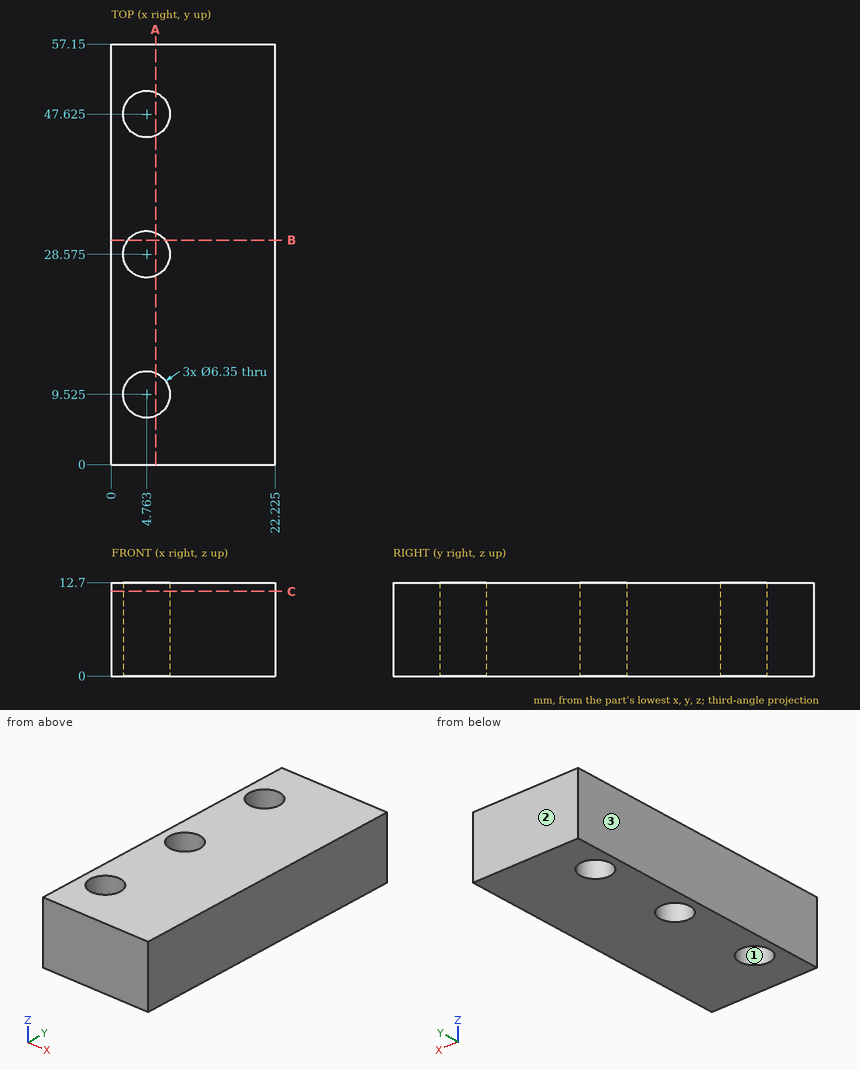
Design review of the part shown in the three views and the two pictorial views. Dimensions are in mm from the part's minimum x, y and z. Coordinates: 2 decimals unless noted, no trailing zeros. Order: outer loops, then holes, each group sorted by start corner. A loop starts at its lowest first (then second) coordinate and runs counter-clockwise, first axis right, second up.
Item 1: For line 1 (Y direction, x = 6.5, z = 4.75); line 2 (X direction, y = 27, z = 12) (1 decimal); line 3 (Y direction, x = 4, z = 7.75), list the stretches that pass through material, from the lowest coordinate up.
Item 2: Take a section at A-A, the plane x = 6. Write out the cut boundary in (y, z), then the cut area to 3 significant figures.
Item 3: The part is to be moulded in two halves that separate along Y. For the marked faces 1, 2 and 3, say which applies: pulls with the +Y half, pulls with the -Y half, needs draft (parallel to the pull), parting line crosses it, or undercut.
Item 4: Take a section at C-C, the plane z = 11.5. Count the separate pieces of the cut face and the enclosed holes in it, then the cut area to 4 significant figures.
Item 5: For pin 1 Ø4 at (x, y) = (4.76, 28.58) entering from +Z, flat-tipped, find the tip position at first contact; note if it passes through.
Item 6: Take a section at B-B, the plane y = 30.5. Write out the cut boundary in (x, z) (1 decimal).
The answers:
1. line 1: y = 0 to 6.87, 12.18 to 25.92, 31.23 to 44.97, 50.28 to 57.15
1. line 2: x = 0 to 2, 7.5 to 22.2
1. line 3: y = 0 to 6.44, 12.61 to 25.49, 31.66 to 44.54, 50.71 to 57.15
2. outline: (0, 0) - (6.6, 0) - (6.6, 12.7) - (0, 12.7) - close; (12.45, 0) - (25.65, 0) - (25.65, 12.7) - (12.45, 12.7) - close; (31.5, 0) - (44.7, 0) - (44.7, 12.7) - (31.5, 12.7) - close; (50.55, 0) - (57.15, 0) - (57.15, 12.7) - (50.55, 12.7) - close
2. area: 503 mm2
3. face 1: undercut
3. face 2: pulls with the +Y half
3. face 3: needs draft
4. separate pieces: 1
4. enclosed holes: 3
4. area: 1,175 mm2
5. pin 1: passes through
6. outline: (0, 0) - (2.2, 0) - (2.2, 12.7) - (0, 12.7) - close; (7.3, 0) - (22.2, 0) - (22.2, 12.7) - (7.3, 12.7) - close
